```python
from build123d import *

# Parameters (mm, degrees)
CROQUIS1_R              = 12.7
SALIENTE_EXTRUIR1_DEPTH = 10
CROQUIS2_R              = 12.7
CROQUIS3_W              = 1.11169581
CROQUIS3_H              = 0.66183921
SALIENTE_EXTRUIR2_DEPTH = 20


with BuildPart() as part:
    # Croquis1 → Saliente-Extruir1 (new body)
    with BuildSketch(Plane.XY):
        Circle(CROQUIS1_R)
    extrude(amount=SALIENTE_EXTRUIR1_DEPTH)

    # Barrer1: sweep along a curve in space
    with BuildLine() as barrer1_path:
        Line((0, 0, 10), (0, 0, 430))
        ThreePointArc((0, 0, 430), (-8.786796564, 0, 451.213203436), (-30, 0, 460))
        Line((-30, 0, 460), (-375, 0, 460))
        ThreePointArc((-375, 0, 460), (-392.67766953, 0, 467.32233047), (-400, 0, 485))
        Line((-400, 0, 485), (-400, 0, 580))
    # Croquis2 → Barrer1 (sweep)
    with BuildSketch(Plane.XY.offset(10)):
        Circle(CROQUIS2_R)
    sweep(path=barrer1_path.line)

    # Croquis3 → Saliente-Extruir2 (add)
    with BuildSketch(Plane(origin=(0, 0, 0), x_dir=(-1, 0, 0), z_dir=(0, 0, -1))):
        with Locations((0, 12.7)):
            Rectangle(CROQUIS3_W, CROQUIS3_H)
    extrude(amount=-SALIENTE_EXTRUIR2_DEPTH)


solid = part.part
```
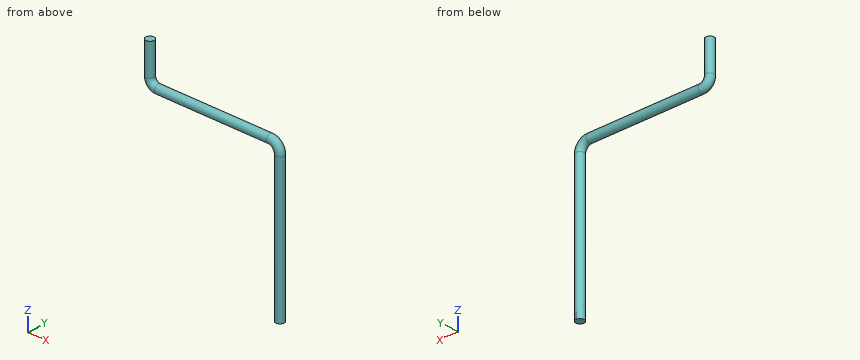
The model under review builds one solid part; all positions refer to its coordinate system, in mm. Round coordinates to 2 decimals unless told otherwise and drop trailing zeros. Write each loop counter-clockwise with the first axis right and the second up, starting at its lowest first coordinate (ties: lowest second). Pieces come first, ordered by that corner, then holes. Notation, with made-up numbers: (43.25, 45.5) -> (54.25, 45.5) arc R16 cw to (54.25, 62.5) -> close; hole circle Ø4 at (-4.75, 17.25). An arc over 180 degrees is marked (long way). Use CSV: the item, a comma, the result in double quotes.
Q1. For pin 1 Ø3 at (x, y) = (-193.5, 3.5) entering from +Z; pin 2 Ø5 at (x, y) = (-276.5, 8.5) entering from +Z, all flat-tipped, find the tip position at first contact; note any pin that passes through.
Checks:
pin 1,"z = 472.54"
pin 2,"z = 471.19"
Q2. Consider section B-B (x = -90). Give the boundary of the cut face in (y, z), then the cut area to 3 significant figures.
Checks:
outline,"circle Ø25.4 at (0, 460)"
area,"507 mm²"
Q3. Consider section C-C (z = 58). Give the boundary of the cut face in (x, y).
Checks:
outline,"circle Ø25.4 at (0, 0)"
Q4. To check wall thickness, follow probe 1 along X at (y, z) = (0, 268); probe 2 along Z at (x, y) = (-196, 0.5); probe 3 along X at (y, z) = (1.75, 204). State the ranges of each line that lie inside material, in increasing order. Write a range as [from, to].
Checks:
probe 1,"[-12.7, 12.7]"
probe 2,"[447.31, 472.69]"
probe 3,"[-12.58, 12.58]"
Q5. Consider section A-A (y = 0). Give the boundary of the cut face in (x, z), then the cut area to 3 significant figures.
Checks:
outline,"(-412.7, 485) arc R37.7 ccw to (-375, 447.3) -> (-30, 447.3) arc R17.3 cw to (-12.7, 430) -> (-12.7, 0) -> (12.7, 0) -> (12.7, 430) arc R42.7 ccw to (-30, 472.7) -> (-375, 472.7) arc R12.3 cw to (-387.3, 485) -> (-387.3, 580) -> (-412.7, 580) -> close"
area,"24,300 mm²"
